```python
from build123d import *

# Parameters (mm, degrees)
SKETCH1_R           = 14.5375
SKETCH1_R_2         = 1.5
SKETCH1_R_3         = 2.5
BOSS_EXTRUDE1_DEPTH = 1.5875
FILLET1_R           = 5
FILLET2_R           = 13
CHAMFER1_SIZE       = 14.249999948
FILLET4_START       = -1
FILLET4_DEPTH       = 4
FILLET4_2_DEPTH     = 1.5875


with BuildPart() as part:
    # Sketch1 → Boss-Extrude1 (new body)
    with BuildSketch(Plane.XY):
        Polygon((14.25, 50), (49.25, 50), (49.25, 0), (63.5, 0), (63.5, -59.087), (0, -59.087), (0, 0), (14.25, 0), align=None)
        with Locations((31.75, -27.337)):
            Circle(SKETCH1_R, mode=Mode.SUBTRACT)
        with Locations((19.25, 45)):
            Circle(SKETCH1_R_2, mode=Mode.SUBTRACT)
        with Locations((19.25, 25)):
            Circle(SKETCH1_R_2, mode=Mode.SUBTRACT)
        with Locations((19.25, 5)):
            Circle(SKETCH1_R_2, mode=Mode.SUBTRACT)
        with Locations(Location((44.25, 5, 0), (0, 0, 180))):
            Circle(SKETCH1_R_2, mode=Mode.SUBTRACT)
        with Locations(Location((44.25, 25, 0), (0, 0, 180))):
            Circle(SKETCH1_R_2, mode=Mode.SUBTRACT)
        with Locations(Location((44.25, 45, 0), (0, 0, 180))):
            Circle(SKETCH1_R_2, mode=Mode.SUBTRACT)
        with Locations((31.75, -51.1495)):
            Circle(SKETCH1_R_3, mode=Mode.SUBTRACT)
        with Locations((11.127770072, -39.24325)):
            Circle(SKETCH1_R_3, mode=Mode.SUBTRACT)
        with Locations((11.127770072, -15.43075)):
            Circle(SKETCH1_R_3, mode=Mode.SUBTRACT)
        with Locations((31.75, -3.5245)):
            Circle(SKETCH1_R_3, mode=Mode.SUBTRACT)
        with Locations((52.372229928, -15.43075)):
            Circle(SKETCH1_R_3, mode=Mode.SUBTRACT)
        with Locations((52.372229928, -39.24325)):
            Circle(SKETCH1_R_3, mode=Mode.SUBTRACT)
    extrude(amount=BOSS_EXTRUDE1_DEPTH)

    # Fillet1
    fillet1_edges = [part.edges().sort_by_distance(p)[0] for p in [
        (14.25, 50, 0.79375),
        (49.25, 50, 0.79375),
    ]]
    fillet(fillet1_edges, radius=FILLET1_R)

    # Fillet2
    fillet2_edges = [part.edges().sort_by_distance(p)[0] for p in [
        (63.5, -59.087, 0.79375),
        (0, -59.087, 0.79375),
    ]]
    fillet(fillet2_edges, radius=FILLET2_R)

    # Chamfer1
    chamfer1_edges = [part.edges().sort_by_distance(p)[0] for p in [
        (49.25, 0, 0.79375),
        (14.25, 0, 0.79375),
    ]]
    chamfer(chamfer1_edges, length=CHAMFER1_SIZE)

    # Fillet4: read off the stored shape, not the designer's step
    # Fillet4 outline → Fillet4 (cut)
    with BuildSketch(Plane.XY.offset(FILLET4_START)):
        with BuildLine():
            ThreePointArc((0, -5.260512294), (0.966729937, -0.400432703), (3.719743879, 3.719743827))
            Line((3.719743879, 3.719743827), (2.6e-08, -2.6e-08))
            Line((2.6e-08, -2.6e-08), (0, -5.260512294))
        make_face()
        with BuildLine():
            Line((63.499999974, -2.6e-08), (59.780256121, 3.719743827))
            ThreePointArc((59.780256121, 3.719743827), (62.533270063, -0.400432703), (63.5, -5.260512294))
            Line((63.5, -5.260512294), (63.499999974, -2.6e-08))
        make_face()
    extrude(amount=FILLET4_DEPTH, mode=Mode.SUBTRACT)

    # Fillet4 2 outline → Fillet4 2 (add)
    with BuildSketch(Plane.XY):
        with BuildLine():
            ThreePointArc((14.25, 19.51051219), (13.283270063, 14.650432599), (10.530256121, 10.530256069))
            Line((10.530256121, 10.530256069), (14.25, 14.249999948))
            Line((14.25, 14.249999948), (14.25, 19.51051219))
        make_face()
        with BuildLine():
            Line((49.25, 14.249999948), (52.969743879, 10.530256069))
            ThreePointArc((52.969743879, 10.530256069), (50.216729937, 14.650432599), (49.25, 19.51051219))
            Line((49.25, 19.51051219), (49.25, 14.249999948))
        make_face()
    extrude(amount=FILLET4_2_DEPTH)


solid = part.part
```
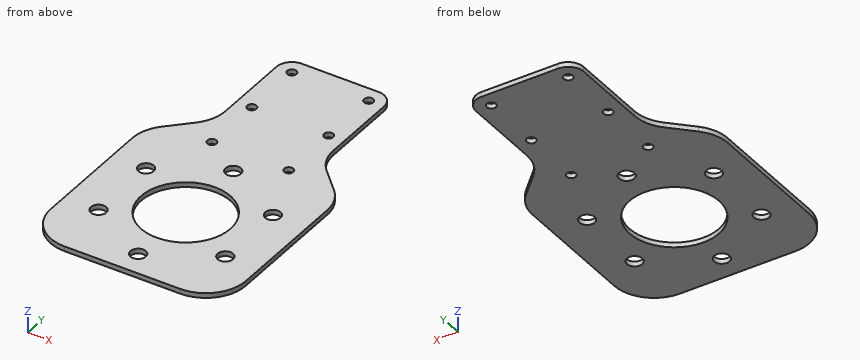
Check sheet for the modelled part. Datum: model origin and axes. Units: mm. Round coordinates to 2 decimals unless told otherwise and drop trailing zeros. Order: outer loops, then holes, each group sorted by start corner. A loop starts at its lowest first (then second) coordinate and runs counter-clockwise, first axis right, second up. Notation, with made-up numbers: (-24, -17.5) - (24, -17.5) arc R16 cw to (24, -6.5) - close; hole circle Ø5 at (64, 2). An arc over 180 degrees is marked (long way). Answer as CSV lines item,"result". Start each with the question number.
1) Depth check by flat-ended pin: pin 1 (3 mm diameter, centred on x = 31.75, y = -3.52, fed in from -Z); pin 2 (3.5 mm diameter, centred on x = 44.25, y = 45, fed in from +Z); pin 3 (0.5 mm diameter, centred on y = 32, z = 1, fed in from -X). Enter the tip coordinate at first touch or a pass-through.
2) Section check A-A (x = 31.75). Record the cut outline in (y, z).
3) Section check C-C (z = 0.9). Give the number of separate pieces and of enclosed holes in the cut face, then the cut area to 3 significant figures.
4) Section check D-D (y = -20). Record the cut outline in (x, z).
5) Section check B-B (y = 5). Record the cut outline in (x, z).
6) Scan lines: probe 1 along Y at (x, z) = (32, 0.5); probe 2 along Y at (x, z) = (13, 0.95); probe 3 along Y at (x, z) = (54, 0.25). Record each from-to range of solid material in increasing order.
Determined:
1,pin 1,"through"
1,pin 2,"z = 1.59"
1,pin 3,"x = 14.25"
2,outline,"(-59.09, 0) - (-53.65, 0) - (-53.65, 1.59) - (-59.09, 1.59) - close; (-48.65, 0) - (-41.87, 0) - (-41.87, 1.59) - (-48.65, 1.59) - close; (-12.8, 0) - (-6.02, 0) - (-6.02, 1.59) - (-12.8, 1.59) - close; (-1.02, 0) - (50, 0) - (50, 1.59) - (-1.02, 1.59) - close"
3,separate pieces,"1"
3,enclosed holes,"13"
3,area,"4,800 mm^2"
4,outline,"(0, 0) - (19.2, 0) - (19.2, 1.59) - (0, 1.59) - close; (44.3, 0) - (63.5, 0) - (63.5, 1.59) - (44.3, 1.59) - close"
5,outline,"(5, 0) - (17.75, 0) - (17.75, 1.59) - (5, 1.59) - close; (20.75, 0) - (42.75, 0) - (42.75, 1.59) - (20.75, 1.59) - close; (45.75, 0) - (58.5, 0) - (58.5, 1.59) - (45.75, 1.59) - close"
6,probe 1,"-59.09 to -53.64, -48.66 to -41.87, -12.8 to -6.01, -1.04 to 50"
6,probe 2,"-59.09 to -40.9, -37.59 to -17.09, -13.77 to 14.02"
6,probe 3,"-58.61 to -41.14, -37.35 to -17.33, -13.53 to 9.5"
